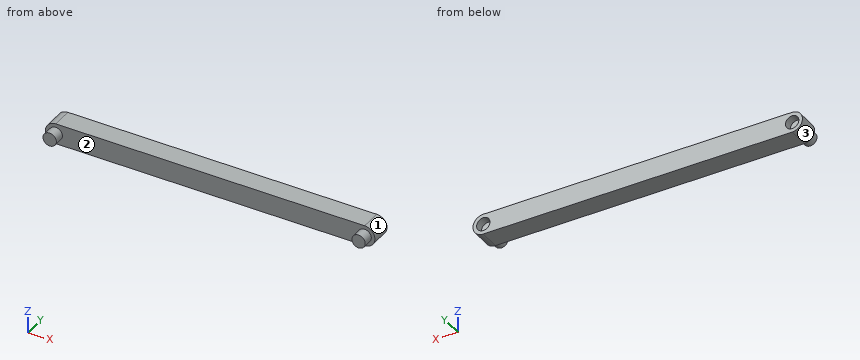
from build123d import *

# Parameters (mm, degrees)
BOSS_EXTRUDE1_DEPTH = 15
SKETCH2_R           = 9.75
CUT_EXTRUDE2_DEPTH  = 241.935676063
BOSS_EXTRUDE2_START = -30
SKETCH2_3_R         = 9.75
BOSS_EXTRUDE2_DEPTH = 30
SKETCH2_4_R         = 9.75
BOSS_EXTRUDE3_DEPTH = 3


with BuildPart() as part:
    # Sketch1 → Boss-Extrude1 (new, symmetric)
    with BuildSketch(Plane(origin=(0, 0, 0), x_dir=(1, 0, 0), z_dir=(0, 1, 0))):
        with BuildLine():
            Line((-225, 15), (225, 15))
            ThreePointArc((225, 15), (240, 0), (225, -15))
            Line((225, -15), (-225, -15))
            ThreePointArc((-225, -15), (-240, 0), (-225, 15))
        make_face()
    extrude(amount=BOSS_EXTRUDE1_DEPTH, both=True)

    # Sketch2 → Cut-Extrude2 (cut, through all)
    with BuildSketch(Plane(origin=(0, 0, 0), x_dir=(1, 0, 0), z_dir=(0, 1, 0))):
        with Locations(Location((-225, 0, 0), (0, 0, 270))):
            Circle(SKETCH2_R)
        with Locations(Location((225, 0, 0), (0, 0, 270))):
            Circle(SKETCH2_R)
    extrude(amount=CUT_EXTRUDE2_DEPTH, mode=Mode.SUBTRACT)

    # Sketch2_3 → Boss-Extrude2 (add)
    with BuildSketch(Plane(origin=(0, 0, 0), x_dir=(1, 0, 0), z_dir=(0, 1, 0)).offset(BOSS_EXTRUDE2_START)):
        with Locations(Location((-225, 0, 0), (0, 0, 270))):
            Circle(SKETCH2_3_R)
        with Locations(Location((225, 0, 0), (0, 0, 270))):
            Circle(SKETCH2_3_R)
    extrude(amount=BOSS_EXTRUDE2_DEPTH)

    # Sketch2_4 → Boss-Extrude3 (add)
    with BuildSketch(Plane(origin=(0, 0, 0), x_dir=(1, 0, 0), z_dir=(0, 1, 0))):
        with Locations(Location((-225, 0, 0), (0, 0, 270))):
            Circle(SKETCH2_4_R)
        with Locations(Location((225, 0, 0), (0, 0, 270))):
            Circle(SKETCH2_4_R)
    extrude(amount=BOSS_EXTRUDE3_DEPTH)


solid = part.part
Read the model definition and answer for the solid it produces. Units are mm, in the model's axes. Face numbers are marked on the shaded views. Coordinates: 2 decimals unless noted, no trailing zeros. Loops run counter-clockwise (first coordinate to the right, second up) from the corner with the lowest first, then second, coordinate; pieces in that order, holes last.
Q1. The part is cut by section C-C on x = 189. Write down the section's boundary in (y, z), and give its area (3 significant figures).
Q2. Consider probe 1 along X at (y, z) = (7, 0); probe 2 along X at (y, z) = (6.5, 9); probe 3 along Z at (x, y) = (-225, 11). Determine where each line is inside the solid, lowest interval first.
Q3. Each of these flat-tipped pins is pushed along its axis until it touches: pin 1 Ø10 at (x, z) = (224.5, 1.5) entering from +Y; pin 2 Ø2 at (y, z) = (-9, -10) entering from -X; pin 3 Ø1.5 at (y, z) = (-24.5, 2.5) entering from +X. Where does it stop, or does it pass through?
Q4. The part is cut by section A-A on z = 0. Write down the section's boundary in (x, y), and give its area (3 significant figures).
Q5. The part is cut by section B-B on y = -19. Write down the section's boundary in (x, z), and give its area (3 significant figures).
Q6. The mould has two halves that part along X. Classify the marked faces 1, 2 and 3: +X half, -X half, draft (parallel to the pull), parting line (faces both ways), or undercut.
Results below:
1. outline: (-15, -15) - (15, -15) - (15, 15) - (-15, 15) - close
1. area: 900 mm2
2. probe 1: x = -240 to -234.75, -215.25 to 215.25, 234.75 to 240
2. probe 2: x = -237 to -228.75, -221.25 to 221.25, 228.75 to 237
2. probe 3: z = -15 to -9.75, 9.75 to 15
3. pin 1: stops at y = 3
3. pin 2: stops at x = -237
3. pin 3: stops at x = 234.59
4. outline: (-240, -15) - (-234.75, -15) - (-234.75, -30) - (-215.25, -30) - (-215.25, -15) - (215.25, -15) - (215.25, -30) - (234.75, -30) - (234.75, -15) - (240, -15) - (240, 15) - (234.75, 15) - (234.75, 3) - (215.25, 3) - (215.25, 15) - (-215.25, 15) - (-215.25, 3) - (-234.75, 3) - (-234.75, 15) - (-240, 15) - close
4. area: 14,500 mm2
5. outline: circle Ø19.5 at (-225, 0); circle Ø19.5 at (225, 0)
5. area: 597 mm2
6. face 1: +X half
6. face 2: undercut
6. face 3: -X half
